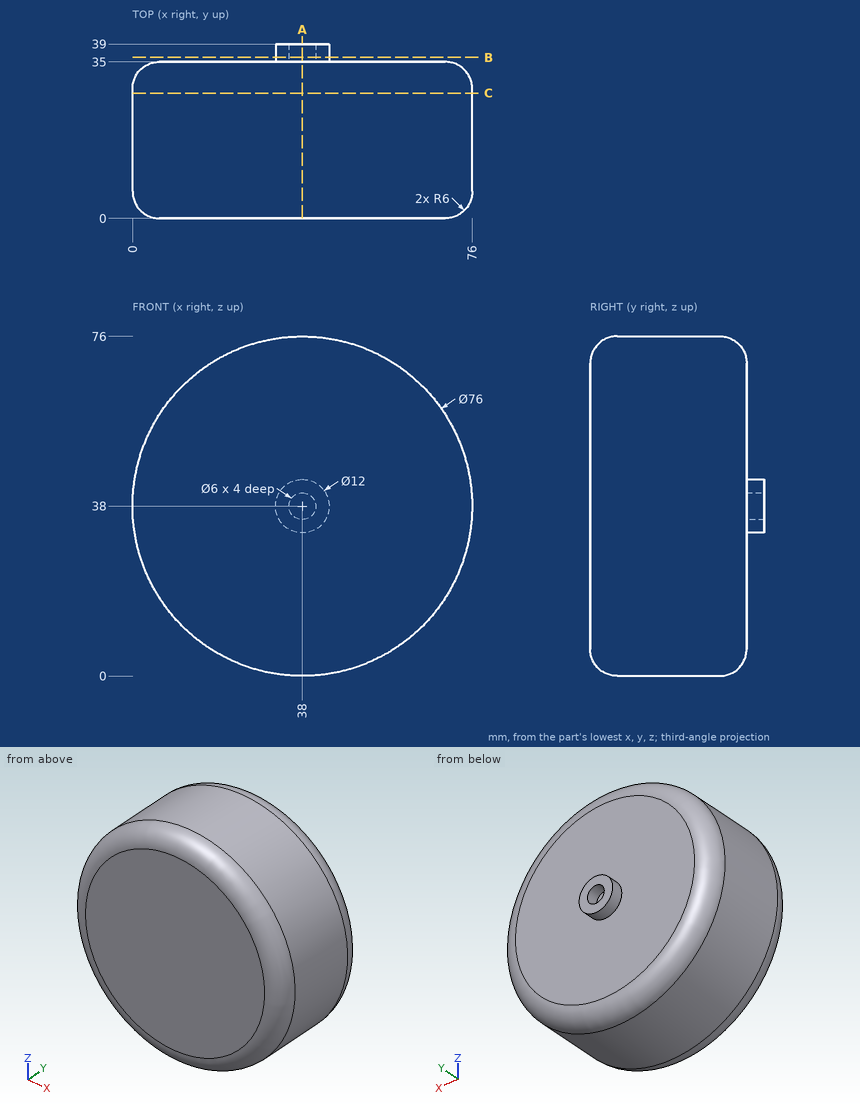
The figure shows three views and two pictorial views of one solid part (mm, origin at its lowest corner). Answer the questions. Round coordinates to 2 decimals unless told otherwise and drop trailing zeros. Write each loop counter-clockwise with the first axis right and the second up, starting at its lowest first coordinate (ties: lowest second). Pieces come first, ordered by that corner, then holes. Notation, with made-up numbers: (8, 25.25) - (40, 25.25) arc R36 ccw to (40, 63.25) - close; hole circle Ø4 at (42, 23.25). An arc over 180 degrees is marked (long way). Answer in a Markdown table with one row per item. Add a question column.
1. Given pin 1 (6.5 mm diameter, centred on x = 39.5, z = 39, fed in from +Y); pin 2 (19 mm diameter, centred on x = 49, z = 26.5, fed in from +Y); pin 3 (6 mm diameter, centred on y = 18.5, z = 23.5, fed in from +X); pin 4 (12 mm diameter, centred on y = 25, z = 43.5, fed in from +X), each flat-ended and moving along its own axis, determine where each tip first touches the part or whether it passes through.
2. Find the intervals of material crossed by line 1 along X through (y, z) = (38.05, 38); line 2 along Y through (x, z) = (26.5, 46); line 3 along X through (y, z) = (3, 64), in increasing order. Write a range as from..to.
3. A cutting plane is placed at B-B, the plane y = 36. Determine the outline of the cut face in (x, z).
4. A cutting plane is placed at A-A, the plane x = 38. Determine the outline of the cut face in (y, z), and give its area (3 significant figures).
5. A cutting plane is placed at C-C, the plane y = 28. Determine the outline of the cut face in (x, z), and give its area (3 significant figures).
Worked out:
| question | item | result |
|---|---|---|
| 1 | pin 1 | y = 39 |
| 1 | pin 2 | y = 35 |
| 1 | pin 3 | x = 74.22 |
| 1 | pin 4 | x = 76 |
| 2 | line 1 | 32..35, 41..44 |
| 2 | line 2 | 0..35 |
| 2 | line 3 | 11.4..64.6 |
| 3 | outline | circle Ø12 at (38, 38); hole circle Ø6 at (38, 38) |
| 4 | outline | (0, 6) arc R6 ccw to (6, 0) - (29, 0) arc R6 ccw to (35, 6) - (35, 32) - (39, 32) - (39, 35) - (35, 35) - (35, 41) - (39, 41) - (39, 44) - (35, 44) - (35, 70) arc R6 ccw to (29, 76) - (6, 76) arc R6 ccw to (0, 70) - close |
| 4 | area | 2,650 mm^2 |
| 5 | outline | circle Ø76 at (38, 38) |
| 5 | area | 4,540 mm^2 |
